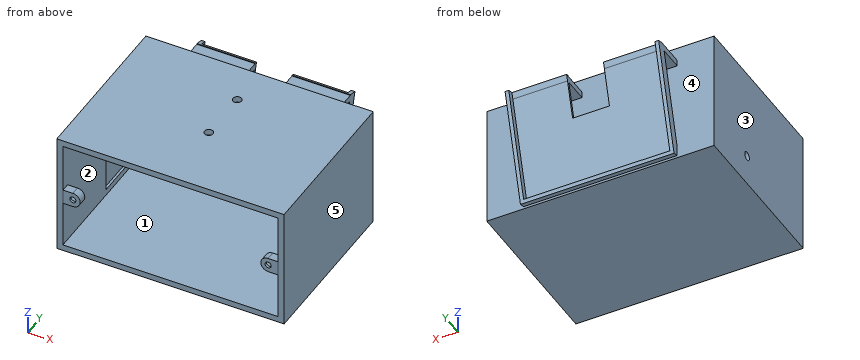
from build123d import *

# Parameters (mm, degrees)
ESBO_O1_W                 = 185
ESBO_O1_H                 = 135
RESSALTO_EXTRUS_O1_DEPTH  = 5
RESSALTO_EXTRUS_O4_START  = 95
ESBO_O1_2_W               = 185
ESBO_O1_2_H               = 135
RESSALTO_EXTRUS_O4_DEPTH  = 5
ESBO_O3_W                 = 185
ESBO_O3_H                 = 100
RESSALTO_EXTRUS_O5_DEPTH  = 5
ESBO_O4_W                 = 100
ESBO_O4_H                 = 135
RESSALTO_EXTRUS_O6_DEPTH  = 5
RESSALTO_EXTRUS_O7_START  = -185
ESBO_O4_3_W               = 100
ESBO_O4_3_H               = 135
RESSALTO_EXTRUS_O7_DEPTH  = 5
ESBO_O8_R                 = 3.5
CORTE_EXTRUS_O1_DEPTH     = 10
RESSALTO_EXTRUS_O10_START = -83.2
ESBO_O10_R                = 2.5
RESSALTO_EXTRUS_O10_DEPTH = 7
CORTE_EXTRUS_O2_START     = -2
CORTE_EXTRUS_O2_DEPTH     = 6
ESBO_O12_R                = 3.5
CORTE_EXTRUS_O4_DEPTH     = 6
ESBO_O13_W                = 30
ESBO_O13_H                = 40
CORTE_EXTRUS_O5_DEPTH     = 2
RESSALTO_EXTRUS_O15_START = -30
RESSALTO_EXTRUS_O15_DEPTH = 125
ESBO_O20_W                = 125
ESBO_O20_H                = 91.931851656
RESSALTO_EXTRUS_O20_DEPTH = 2
RESSALTO_EXTRUS_O21_DEPTH = 5
ESBO_O22_W                = 30
ESBO_O22_H                = 35
CORTE_EXTRUS_O6_DEPTH     = 2
ESBO_O23_W                = 30
ESBO_O23_H                = 21.223161699
CORTE_EXTRUS_O7_DEPTH     = 5


with BuildPart() as part:
    # Esbo_o1 → Ressalto-extrus_o1 (new body)
    with BuildSketch(Plane.XY):
        with Locations((13.448247946, -22.785875217)):
            Rectangle(ESBO_O1_W, ESBO_O1_H)
    extrude(amount=RESSALTO_EXTRUS_O1_DEPTH)



with BuildPart() as body_2:
    # Esbo_o1_2 → Ressalto-extrus_o4 (new body)
    with BuildSketch(Plane.XY.offset(RESSALTO_EXTRUS_O4_START)):
        with Locations((13.448247946, -22.785875217)):
            Rectangle(ESBO_O1_2_W, ESBO_O1_2_H)
    extrude(amount=RESSALTO_EXTRUS_O4_DEPTH)


with BuildPart() as part_1:
    add(part.part)

    add(body_2.part)  # Ressalto-extrus_o5 merges body 2
    # Esbo_o3 → Ressalto-extrus_o5 (add)
    with BuildSketch(Plane(origin=(0, 44.714124783, 0), x_dir=(1, 0, 0), z_dir=(0, 1, 0))):
        with Locations((13.448247946, -50)):
            Rectangle(ESBO_O3_W, ESBO_O3_H)
    extrude(amount=-RESSALTO_EXTRUS_O5_DEPTH)

    # Esbo_o4 → Ressalto-extrus_o6 (add)
    with BuildSketch(Plane.ZY.offset(79.051752054)):
        with Locations((50, -22.785875217)):
            Rectangle(ESBO_O4_W, ESBO_O4_H)
    extrude(amount=-RESSALTO_EXTRUS_O6_DEPTH)

    # Esbo_o4_3 → Ressalto-extrus_o7 (add)
    with BuildSketch(Plane.ZY.offset(79.051752054).offset(RESSALTO_EXTRUS_O7_START)):
        with Locations((50, -22.785875217)):
            Rectangle(ESBO_O4_3_W, ESBO_O4_3_H)
    extrude(amount=RESSALTO_EXTRUS_O7_DEPTH)

    # Esbo_o8 → Corte-extrus_o1 (cut)
    with BuildSketch(Plane.XY.offset(100)):
        with Locations((13.448247946, 10.836303666)):
            Circle(ESBO_O8_R)
        with Locations((13.448247946, -32.163696334)):
            Circle(ESBO_O8_R)
    extrude(amount=-CORTE_EXTRUS_O1_DEPTH, mode=Mode.SUBTRACT)

    # Esbo_o10 → Ressalto-extrus_o10 (add)
    # profile 1 of 2: a face of its own
    with BuildSketch(Plane(origin=(0, 0, 0), x_dir=(1, 0, 0), z_dir=(0, 1, 0)).offset(RESSALTO_EXTRUS_O10_START)):
        with BuildLine():
            Line((100.948247946, -55), (92.948247946, -55))
            ThreePointArc((92.948247946, -55), (86.948247946, -49), (92.948247946, -43))
            Line((92.948247946, -43), (100.948247946, -43))
            Line((100.948247946, -43), (100.948247946, -55))
        make_face()
        with Locations(Location((92.948247946, -49, 0), (0, 0, 270))):
            Circle(ESBO_O10_R, mode=Mode.SUBTRACT)
    # profile 2 of 2: a face of its own
    with BuildSketch(Plane(origin=(0, 0, 0), x_dir=(1, 0, 0), z_dir=(0, 1, 0)).offset(RESSALTO_EXTRUS_O10_START)):
        with BuildLine():
            Line((-74.051752054, -43), (-74.051752054, -55))
            Line((-74.051752054, -55), (-66.051752054, -55))
            ThreePointArc((-66.051752054, -55), (-60.051752054, -49), (-66.051752054, -43))
            Line((-66.051752054, -43), (-74.051752054, -43))
        make_face()
        with Locations(Location((-66.051752054, -49, 0), (0, 0, 90))):
            Circle(ESBO_O10_R, mode=Mode.SUBTRACT)
    extrude(amount=-RESSALTO_EXTRUS_O10_DEPTH)

    # Esbo_o11 → Corte-extrus_o2 (cut)
    with BuildSketch(Plane.XZ.offset(90.2).offset(CORTE_EXTRUS_O2_START)):
        Polygon((-61.75961018, 51.564667257), (-66.126748114, 53.999437527), (-70.418889987, 51.43477027), (-70.343893927, 46.435332743), (-65.976755993, 44.000562473), (-61.68461412, 46.56522973), align=None)
        Polygon((88.581110013, 46.56522973), (88.656106073, 51.564667257), (93.023244007, 53.999437527), (97.31538588, 51.43477027), (97.24038982, 46.435332743), (92.873251886, 44.000562473), align=None)
    extrude(amount=-CORTE_EXTRUS_O2_DEPTH, mode=Mode.SUBTRACT)

    # Esbo_o12 → Corte-extrus_o4 (cut)
    with BuildSketch(Plane.ZY.offset(79.051752054)):
        with Locations(Location((25, -5.285875217, 0), (0, 0, 270))):
            Circle(ESBO_O12_R)
    extrude(amount=-CORTE_EXTRUS_O4_DEPTH, mode=Mode.SUBTRACT)

    # Esbo_o13 → Corte-extrus_o5 (cut)
    with BuildSketch(Plane(origin=(-74.051752054, 0, 0), x_dir=(0, 0, -1), z_dir=(1, 0, 0))):
        with Locations((-25, -5.285875217)):
            Rectangle(ESBO_O13_W, ESBO_O13_H)
    extrude(amount=-CORTE_EXTRUS_O5_DEPTH, mode=Mode.SUBTRACT)

    # Esbo_o15 → Ressalto-extrus_o15 (add)
    with BuildSketch(Plane(origin=(105.948247946, 0, 0), x_dir=(0, 0, -1), z_dir=(1, 0, 0)).offset(RESSALTO_EXTRUS_O15_START)):
        Polygon((-83.93332437, 66.66809288), (-83.93332437, 44.714124783), (-88.93332437, 44.714124783), (-88.93332437, 68.007838843), align=None)
    extrude(amount=-RESSALTO_EXTRUS_O15_DEPTH)

    # Esbo_o20 → Ressalto-extrus_o20 (add)
    with BuildSketch(Plane(origin=(0, 41.218846376, -11.044556599), x_dir=(1, 0, 0), z_dir=(0, 0.9659258262890665, -0.25881904510252707))):
        with Locations((13.448247946, -57.538792907)):
            Rectangle(ESBO_O20_W, ESBO_O20_H)
    extrude(amount=-RESSALTO_EXTRUS_O20_DEPTH)

    # Esbo_o21 → Ressalto-extrus_o21 (add)
    with BuildSketch(Plane(origin=(0, 41.218846376, -11.044556599), x_dir=(1, 0, 0), z_dir=(0, 0.9659258262890684, -0.2588190451025204))):
        Polygon((75.948247946, -13.504718735), (-49.051752054, -13.504718735), (-49.051752054, -16.504718735), (-49.051752054, -103.504718735), (-46.051752054, -103.504718735), (-46.051752054, -16.504718735), (72.948247946, -16.504718735), (72.948247946, -103.504718735), (75.948247946, -103.504718735), (75.948247946, -16.504718735), align=None)
    extrude(amount=RESSALTO_EXTRUS_O21_DEPTH)

    # Esbo_o22 → Corte-extrus_o6 (cut)
    with BuildSketch(Plane(origin=(0, 41.218846376, -11.044556599), x_dir=(1, 0, 0), z_dir=(0, 0.9659258262890684, -0.2588190451025204))):
        with Locations((13.448247946, -86.004718735)):
            Rectangle(ESBO_O22_W, ESBO_O22_H)
    extrude(amount=-CORTE_EXTRUS_O6_DEPTH, mode=Mode.SUBTRACT)

    # Esbo_o23 → Corte-extrus_o7 (cut)
    with BuildSketch(Plane.XY.offset(88.93332437)):
        with Locations((13.448247946, 55.325705633)):
            Rectangle(ESBO_O23_W, ESBO_O23_H)
    extrude(amount=-CORTE_EXTRUS_O7_DEPTH, mode=Mode.SUBTRACT)


solid = part_1.part
Input: part model. Units: mm. Frame: model coordinates. Face numbers are marked on the shaded views. A direction names the side the tool comes from. Round coordinates to 2 decimals unless told otherwise and drop trailing zeros. Order: outer loops, then holes, each group sorted by start corner. A loop starts at its lowest first (then second) coordinate and runs counter-clockwise, first axis right, second up.
1. Cut plane D-D, the plane x = 14.5. Output: boundary loops of the cut face in (y, z), then the cut area to 3 significant figures.
The answers:
outline: (-90.29, 0) - (44.71, 0) - (44.71, 2) - (49.54, 0.71) - (50.32, 3.6) - (45.49, 4.9) - (58.95, 55.13) - (57.02, 55.64) - (44.71, 9.73) - (44.71, 100) - (14.17, 100) - (14.17, 95) - (39.71, 95) - (39.71, 5) - (-90.29, 5) - close; (-90.29, 95) - (-35.5, 95) - (-35.5, 100) - (-90.29, 100) - close; (-28.83, 95) - (7.5, 95) - (7.5, 100) - (-28.83, 100) - close
area: 1,850 mm2
2. Set-up query: the marked faces 1, 2 and 3. Return all of +Z, -Z, +X, -X, +Y, -Y with unobstructed straight access to the full face (end or side cutting, diameter ignored); none if empty.
The answers:
face 1: -Y
face 2: none
face 3: +Z, -Z, -X, +Y, -Y
3. Cut plane C-C, the plane x = 36. Output: boundary loops of the cut face in (y, z), then the cut area to 3 significant figures.
The answers:
outline: (-90.29, 0) - (44.71, 0) - (44.71, 2) - (49.54, 0.71) - (50.32, 3.6) - (45.49, 4.9) - (68.01, 88.93) - (66.08, 89.45) - (65.94, 88.93) - (44.71, 88.93) - (44.71, 100) - (-90.29, 100) - (-90.29, 95) - (39.71, 95) - (39.71, 5) - (-90.29, 5) - close; hole (44.71, 9.73) - (64.6, 83.93) - (44.71, 83.93) - close
area: 2,090 mm2
4. Cut plane B-B, the plane z = 25. Output: boundary loops of the cut face in (x, y).
The answers:
outline: (-79.05, -90.29) - (-74.05, -90.29) - (-74.05, -25.29) - (-76.05, -25.29) - (-76.05, -8.79) - (-79.05, -8.79) - close; (-79.05, -1.79) - (-76.05, -1.79) - (-76.05, 14.71) - (-74.05, 14.71) - (-74.05, 39.71) - (100.95, 39.71) - (100.95, -90.29) - (105.95, -90.29) - (105.95, 44.71) - (-79.05, 44.71) - close; (-49.05, 48.81) - (75.95, 48.81) - (75.95, 56.05) - (72.95, 56.05) - (72.95, 50.88) - (-46.05, 50.88) - (-46.05, 56.05) - (-49.05, 56.05) - close
5. Pin query (flat end, axial travel): P1, Ø6, axis at x = -64.5, z = 47, coming from the +Y side; P2, Ø14, axis at y = 53, z = 63.5, coming from the +X side; P3, Ø10, axis at x = 69.5, z = 21.5, coming from the -Y side. Return the tip coordinate at first contact, or that it passes through.
The answers:
P1: stops at y = 44.71
P2: stops at x = 75.95
P3: stops at y = 39.71
6. Mould query, pull axis Y, two halves, no side actions, for the marked faces 4 and 5. Classes: released by +Y, released by -Y, zero draft, split by the parting line, or undercut.
The answers:
face 4: undercut
face 5: zero draft
7. Cut plane A-A, the plane y = -38. Output: boundary loops of the cut face in (x, z).
The answers:
outline: (-79.05, 0) - (105.95, 0) - (105.95, 100) - (-79.05, 100) - close; hole (-74.05, 5) - (100.95, 5) - (100.95, 95) - (-74.05, 95) - close
8. Material intervals for line 1 (X direction, y = -89, z = 49); line 2 (Z direction, x = -9, y = 23); line 3 (X direction, y = -68, z = 53), sorted ascending.
The answers:
line 1: x = -79.05 to -68.55, -63.55 to -60.05, 86.95 to 90.45, 95.45 to 105.95
line 2: z = 0 to 5, 95 to 100
line 3: x = -79.05 to -74.05, 100.95 to 105.95
